```python
from build123d import *

# Parameters (mm, degrees)
F0_W          = 152.4
F0_H          = 76.2
F0_W_2        = 139.7
F0_H_2        = 63.5
F1_DEPTH      = 19.05
F2_R          = 9.525
F3_DEPTH      = 38.1
F3_DEPTH_BACK = 38.1
F4_R          = 6.35


with BuildPart() as f1:
    # F0 (on Top) → F1 (new body, symmetric)
    with BuildSketch(Plane.XY):
        Rectangle(F0_W, F0_H)
        Rectangle(F0_W_2, F0_H_2, mode=Mode.SUBTRACT)
    extrude(amount=F1_DEPTH, both=True)

    # F2 (on Front) → F3 (cut, two sides)
    with BuildSketch(Plane.XZ) as f3_sk:
        Circle(F2_R)
    extrude(amount=F3_DEPTH, mode=Mode.SUBTRACT)
    extrude(f3_sk.sketch, amount=-F3_DEPTH_BACK, mode=Mode.SUBTRACT)

    # F4
    f4_edges = [f1.edges().sort_by_distance(p)[0] for p in [
        (-69.85, -31.75, 0),
        (-69.85, 31.75, 0),
        (69.85, 31.75, 0),
        (69.85, -31.75, 0),
        (-76.2, -38.1, 0),
        (76.2, -38.1, 0),
        (76.2, 38.1, 0),
        (-76.2, 38.1, 0),
    ]]
    fillet(f4_edges, radius=F4_R)


solid = f1.part
```
Geometry check sheet. Reference: the model listing, model coordinates, mm. A direction names the side the tool comes from. Give positions to 0.01 mm unless a question says otherwise; leave off trailing zeros. Order: outer loops, then holes, each group sorted by start corner. A loop starts at its lowest first (then second) coordinate and runs counter-clockwise, first axis right, second up.
1. Thickness scan on L1, parallel to Y at x = -54, z = 13; L2, parallel to X at y = -10, z = -15.5; L3, parallel to Z at x = 0, y = -34.25 (3 decimals). Record the ranges inside material, lowest first.
2. Section check D-D, the plane z = 0. Enter the section's corners in (x, y) (3 decimals), and give its area (3 significant figures).
3. Release check for a two-part mould opening along Y. For faces 1 (the face through (69.85, 0, 0)), 2 (the face through (-76.2, 0, 0)), 3 (the face through (-74.39, -36.19, 0.27)) record: pulls with the +Y half, pulls with the -Y half, needs draft (parallel to the pull), parting line crosses it, or undercut.
4. Section check C-C, the plane z = -11.5. Enter the section's corners in (x, y), and give its area (3 significant figures).
5. Section check B-B, the plane x = 56.5. Enter the section's corners in (y, z).
6. Access from +Z, -Z, +X, -X, +Y, -Y to the whole of each face (thin tool, end or side, straight path). Record for faces 4 (the face through (67.94, -29.94, -0.27)), 5 (the face through (0, -34, 19.05)).
7. Section check A-A, the plane y = 6.5. Enter the section's corners in (x, z).
Values follow:
1. L1: y = -38.1 to -31.75, 31.75 to 38.1
1. L2: x = -76.2 to -69.85, 69.85 to 76.2
1. L3: z = -19.05 to -9.525, 9.525 to 19.05
2. outline: (-76.2, -31.75) arc R6.35 ccw to (-69.85, -38.1) - (-9.525, -38.1) - (-9.525, -31.75) - (-63.5, -31.75) arc R6.35 cw to (-69.85, -25.4) - (-69.85, 25.4) arc R6.35 cw to (-63.5, 31.75) - (-9.525, 31.75) - (-9.525, 38.1) - (-69.85, 38.1) arc R6.35 ccw to (-76.2, 31.75) - close; (9.525, -38.1) - (69.85, -38.1) arc R6.35 ccw to (76.2, -31.75) - (76.2, 31.75) arc R6.35 ccw to (69.85, 38.1) - (9.525, 38.1) - (9.525, 31.75) - (63.5, 31.75) arc R6.35 cw to (69.85, 25.4) - (69.85, -25.4) arc R6.35 cw to (63.5, -31.75) - (9.525, -31.75) - close
2. area: 2,500 mm2
3. face 1: undercut
3. face 2: needs draft
3. face 3: pulls with the -Y half
4. outline: (-76.2, -31.75) arc R6.35 ccw to (-69.85, -38.1) - (69.85, -38.1) arc R6.35 ccw to (76.2, -31.75) - (76.2, 31.75) arc R6.35 ccw to (69.85, 38.1) - (-69.85, 38.1) arc R6.35 ccw to (-76.2, 31.75) - close; hole (-69.85, -25.4) arc R6.35 ccw to (-63.5, -31.75) - (63.5, -31.75) arc R6.35 ccw to (69.85, -25.4) - (69.85, 25.4) arc R6.35 ccw to (63.5, 31.75) - (-63.5, 31.75) arc R6.35 ccw to (-69.85, 25.4) - close
4. area: 2,740 mm2
5. outline: (-38.1, -19.05) - (-31.75, -19.05) - (-31.75, 19.05) - (-38.1, 19.05) - close; (31.75, -19.05) - (38.1, -19.05) - (38.1, 19.05) - (31.75, 19.05) - close
6. face 4: +Z, -Z
6. face 5: +Z, +X, -X, +Y, -Y
7. outline: (-76.2, -19.05) - (-69.85, -19.05) - (-69.85, 19.05) - (-76.2, 19.05) - close; (69.85, -19.05) - (76.2, -19.05) - (76.2, 19.05) - (69.85, 19.05) - close
